```python
from build123d import *

# Parameters (mm, degrees)
BOSS_EXTRUDE1_DEPTH = 40
BOSS_EXTRUDE2_DEPTH = 20


with BuildPart() as part:
    # Sketch1 → Boss-Extrude1 (new body)
    with BuildSketch(Plane.XY):
        Polygon((0, 10), (0, 0), (50, 0), (50, 18), (40, 18), (40, 8), (25, 8), (25, 18), (4.8, 18), align=None)
    extrude(amount=BOSS_EXTRUDE1_DEPTH)

    # Sketch1<3> → Boss-Extrude2 (add)
    with BuildSketch(Plane.XY):
        Polygon((40, 18), (50, 18), (50, 35), (15, 35), (4.8, 18), (25, 18), (25, 28.078689743), (40, 28.078689743), align=None)
    extrude(amount=BOSS_EXTRUDE2_DEPTH)


solid = part.part
```
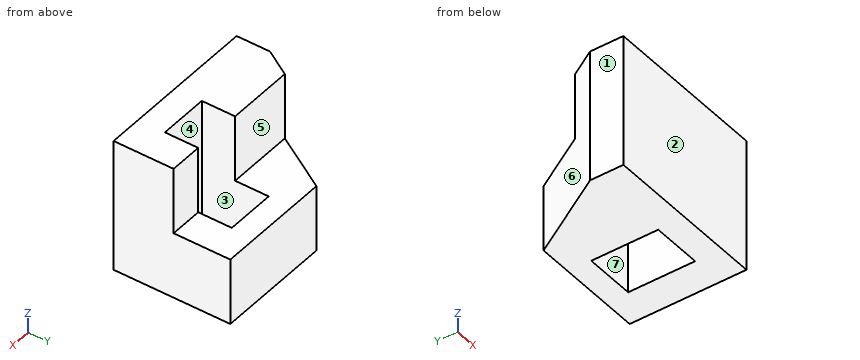
The model under review builds one solid part; all positions refer to its coordinate system, in mm. Face numbers are marked on the shaded views. A direction names the side the tool comes from. Give positions to 0.01 mm unless a question says otherwise; leave off trailing zeros. Loops run counter-clockwise (first coordinate to the right, second up) from the corner with the lowest first, then second, coordinate; pieces in that order, holes last. Notation, with made-up numbers: (25, 6.25) - (53, 6.25) arc R29 ccw to (53, 29.25) - close; hole circle Ø11 at (63.25, 18). An arc over 180 degrees is marked (long way). Answer as a JSON object with one key per item and string values.
Q1. Add section A-A on y = 25. State the section outline as (x, z) points.
Worked out:
{"outline": "(9, 0) - (25, 0) - (25, 20) - (9, 20) - close; (40, 0) - (50, 0) - (50, 20) - (40, 20) - close"}
Q2. Add section B-B on z = 3. State the section outline as (x, y) points, plus the area to 3 significant figures.
Worked out:
{"outline": "(0, 0) - (50, 0) - (50, 35) - (15, 35) - (0, 10) - close; hole (25, 8) - (40, 8) - (40, 28.08) - (25, 28.08) - close", "area": "1,260 mm^2"}
Q3. Add section C-C on x = 37. State the section outline as (y, z) points, plus the area to 3 significant figures.
Worked out:
{"outline": "(0, 0) - (8, 0) - (8, 40) - (0, 40) - close; (28.08, 0) - (35, 0) - (35, 20) - (28.08, 20) - close", "area": "458 mm^2"}
Q4. To check wall thickness, follow line 1 along X through (y, z) = (10, 27.5); line 2 along Y through (x, z) = (25.5, 5.5); line 3 along X through (y, z) = (13, 10). State the ranges of each line that lie inside material, in increasing order.
Worked out:
{"line 1": "x = 0 to 25, 40 to 50", "line 2": "y = 0 to 8, 28.08 to 35", "line 3": "x = 1.8 to 25, 40 to 50"}
Q5. For the marked faces 5, 6 and 7, list the 3-axis set-ups (+Z, -Z, +X, -X, +Y, -Y) from which the entire face can be reached by the end or side of a thin tool; tool diameter is ignored.
Worked out:
{"face 5": "+Z, +X, -X, +Y", "face 6": "+Z, -Z, -X, +Y", "face 7": "+Z, -Z"}
Q6. Insertion check: pin 1 (6 mm diameter, centred on x = 17, z = 28, fed in from +Y); pin 2 (6 mm diameter, centred on y = 19.5, z = 31, fed in from -X); pin 3 (1.5 mm diameter, centred on x = 23.5, y = 21.5, fed in from +Z). Each pin has a flat end and moves straight along its axis. Give the tip position at first contact, or say it passes through.
Worked out:
{"pin 1": "stops at y = 18", "pin 2": "stops at x = 3.9", "pin 3": "stops at z = 20"}
Q7. Add section D-D on z = 31.5. State the section outline as (x, y) points.
Worked out:
{"outline": "(0, 0) - (50, 0) - (50, 18) - (40, 18) - (40, 8) - (25, 8) - (25, 18) - (4.8, 18) - (0, 10) - close"}
Q8. Mouldability with a two-part tool opening along X and no side actions: class the marked faces 1, 2, 3 and 4 as +X half, -X half, draft (parallel to the pull), parting line (faces both ways), or undercut.
Worked out:
{"face 1": "-X half", "face 2": "draft", "face 3": "undercut", "face 4": "undercut"}
